Check sheet for the modelled part. Datum: model origin and axes. Units: mm. Face numbers are marked on the shaded views. Give positions to 0.01 mm unless a question says otherwise; leave off trailing zeros. Write each loop counter-clockwise with the first axis right and the second up, starting at its lowest first coordinate (ties: lowest second). Pieces come first, ordered by that corner, then holes. Notation, with made-up numbers: M -25,-1 L -18,-1 A25 cw -18,24 Z; hole C -31.5,-12.5 d4. An arc over 180 degrees is marked long. One line per item, written item: value. Start each with the question number.
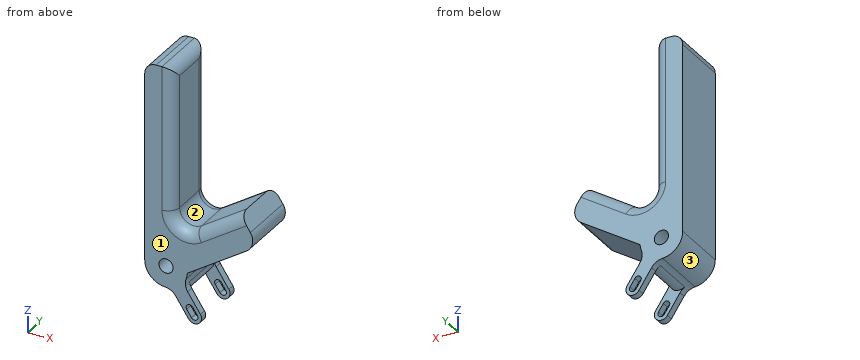
from build123d import *

# Parameters (mm, degrees)
F0_R        = 3.175
F1_DEPTH    = 25.4
F2_R        = 5.08
F3_W        = 19.05
F3_H        = 15.7622399921
F4_DEPTH    = 6.35
F5_T1_DEPTH = 19.05


# Not quite as in the source:
# - a fillet or chamfer that OpenCascade refuses, or shapes differently, is made with other operations: its cross-section is extruded or revolved along the edge and cut away or added


with BuildPart() as f1:
    # F0 (on Front) → F1 (new body)
    with BuildSketch(Plane.XZ):
        with BuildLine():
            ThreePointArc((-0.6915815922, -12.1052896192), (-1.7090267403, -9.3705639378), (-1.3960508414, -6.4695356255))
            ThreePointArc((-1.3960508414, -6.4695356255), (-1.0364150689, -5.1594737521), (-0.8668126136, -3.8115735302))
            Line((-0.8668126136, -3.8115735302), (25.5427133598, 13.7947321605))
            ThreePointArc((25.5427133598, 13.7947321605), (28.2470591636, 17.8329108842), (27.3038968609, 22.6005956999))
            Line((27.3038968609, 22.6005956999), (22.778728087, 29.3883661936))
            Line((22.778728087, 29.3883661936), (2.6693062503, 15.9821192025))
            ThreePointArc((2.6693062503, 15.9821192025), (-3.8493348951, 15.6670107863), (-7.2030337688, 21.2656427228))
            Line((-7.2030337688, 21.2656427228), (-7.2030337688, 85.6005759959))
            Line((-7.2030337688, 85.6005759959), (-19.9030337688, 85.6005759959))
            Line((-19.9030337688, 85.6005759959), (-19.9030337688, -3.2994240041))
            ThreePointArc((-19.9030337688, -3.2994240041), (-17.2975054683, -9.8451505795), (-10.9063857057, -12.8097588684))
            ThreePointArc((-10.9063857057, -12.8097588684), (-8.1081380718, -13.6366381587), (-5.9751009613, -15.6276358652))
            Line((-5.9751009613, -15.6276358652), (-0.3197934533, -24.1105971271))
            ThreePointArc((-0.3197934533, -24.1105971271), (4.0831393542, -24.9911836886), (4.9637259157, -20.5882508811))
            Line((4.9637259157, -20.5882508811), (-0.6915815922, -12.1052896192))
        make_face()
        with Locations((-10.3780337688, -3.2994240041)):
            Circle(F0_R, mode=Mode.SUBTRACT)
        with BuildLine():
            ThreePointArc((3.6428460735, -21.4688374426), (3.2025527927, -23.6703038464), (1.0010863889, -23.2300105656))
            Line((1.0010863889, -23.2300105656), (-1.131874873, -20.0305686727))
            ThreePointArc((-1.131874873, -20.0305686727), (-0.6915815922, -17.829102269), (1.5098848115, -18.2693955497))
            Line((1.5098848115, -18.2693955497), (3.6428460735, -21.4688374426))
        make_face(mode=Mode.SUBTRACT)
    extrude(amount=F1_DEPTH)

    # F2
    f2_edges = [f1.edges().sort_by_distance(p)[0] for p in [
        (-7.203034, -25.4, 53.433109),
        (-7.203034, 0, 53.433109),
        (-7.203034, -12.7, 85.600576),
        (-19.903034, -12.7, 85.600576),
    ]]
    fillet(f2_edges, radius=F2_R)

    # F3 (on face) → F4 (cut, through all)
    with BuildSketch(Plane(origin=(-6.0658440035, 0, -4.0438960023), x_dir=(0, 1, 0), z_dir=(0.8320502943, 0, 0.5547001962))):
        with Locations((-12.7, -17.5697093418)):
            Rectangle(F3_W, F3_H)
    extrude(amount=-F4_DEPTH, mode=Mode.SUBTRACT)

    # F5: fillet of radius 5.08 on 6 edges, made by hand

    # F5_s2 → F5_t1 (cut)
    with BuildSketch(Plane.XZ.offset(3.175)):
        with BuildLine():
            ThreePointArc((-1.706559996, -9.3900529107), (-2.1228958796, -12.1426914098), (-3.9274812175, -14.262556036))
            Line((-3.9274812175, -14.262556036), (-0.6915815922, -12.1052896192))
            ThreePointArc((-0.6915815922, -12.1052896192), (-1.3560793604, -10.8063623925), (-1.706559996, -9.3900529107))
        make_face()
        with BuildLine():
            ThreePointArc((-8.0910969984, -13.6464109123), (-5.3900707363, -14.3208079809), (-2.739201336, -13.4703694484))
            Line((-2.739201336, -13.4703694484), (-5.9751009613, -15.6276358652))
            ThreePointArc((-5.9751009613, -15.6276358652), (-6.9185346443, -14.5146659151), (-8.0910969984, -13.6464109123))
        make_face()
    extrude(amount=F5_T1_DEPTH, mode=Mode.SUBTRACT)


solid = f1.part
1) Cross-section at B-B (z = 62). Record the boundary of the cut face in (x, y), plus the area to 3 significant figures.
2) Draft check along X on the marked faces 1, 2 and 3. Enter one of: released by +X, released by -X, zero draft, split by the parting line, or undercut.
3) Gauge pin test, flat ends, axial feed: pin 1 (8 mm diameter, centred on x = -7.5, z = 25.5, fed in from +Y); pin 2 (3 mm diameter, centred on y = -11, z = 13.5, fed in from +X); pin 3 (8 mm diameter, centred on y = -22.5, z = -10, fed in from -X); pin 4 (7 mm diameter, centred on x = -1, z = -21, fed in from +Y). Record the tip position at first contact, or that the pin passes through.
4) Material ranges on L1, parallel to Y at x = 23, z = 24; L2, parallel to Z at x = -12, y = -7.75; L3, parallel to X at y = -7.75, z = 33.5, recorded low to high. Write a range as from..to.
Data:
1. outline: M -19.9,-25.4 L -12.28,-25.4 A5.08 ccw -7.2,-20.32 L -7.2,-5.08 A5.08 ccw -12.28,0 L -19.9,0 Z
1. area: 312 mm2
2. face 1: zero draft
2. face 2: undercut
2. face 3: released by -X
3. pin 1: stops at y = -0.06
3. pin 2: stops at x = 26.89
3. pin 3: stops at x = -19.51
3. pin 4: stops at y = 0
4. L1: y = -25.38..-0.02
4. L2: z = -12.69..-6.03, -0.57..85.59
4. L3: x = -19.9..-7.2
